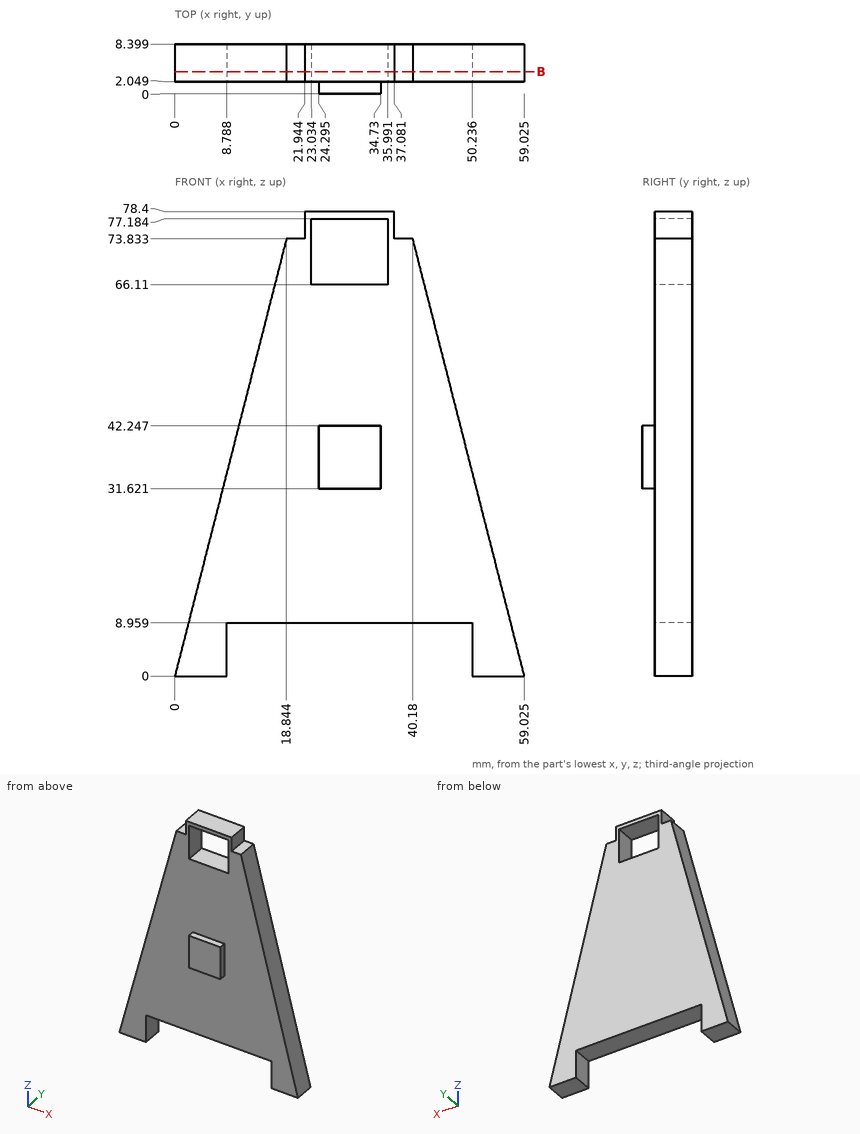
Check sheet for the drawn part. Datum: minimum x, y, z corner. Units: mm. Give positions to 0.01 mm unless a question says otherwise; leave off trailing zeros. Loops run counter-clockwise (first coordinate to the right, second up) from the corner with the lowest first, then second, coordinate; pieces in that order, holes last. Notation, with made-up numbers: (-15.5, 86.25) - (8.5, 86.25) arc R23 ccw to (8.5, 122.25) - close; hole circle Ø8 at (85.5, 31.25). An arc over 180 degrees is marked (long way). Write each question's results on one line, items separated by ' | '.
1) Depth check by flat-ended pin: P1, Ø2.5, axis at y = 3.5, z = 77, coming from the -X side; P2, Ø3.5, axis at y = 5.5, z = 76, coming from the +X side; P3, Ø1.6, axis at x = 29.5, y = 1.5, coming from the -Z side; P4, Ø17.5, axis at x = 26.5, z = 45, coming from the -Y side. Enter the tip coordinate at first touch or a pass-through.
Solution:
P1: x = 21.94 | P2: x = 37.08 | P3: z = 8.96 | P4: y = 0
2) Material ranges on L1, parallel to Z at x = 35, y = 5.75 (1 decimal); L2, parallel to Y at x = 4, z = 15; L3, parallel to Z at x = 40, y = 3.5, recorded low to high. Write a range as from..to.
Solution:
L1: 9..66.1, 77.2..78.4 | L2: 2.05..8.4 | L3: 8.96..73.83
3) Sectioned sample at B-B on y = 3.75. Record the boundary of the cut face in (x, z) (1 decimal).
Solution:
outline: (0, 0) - (8.8, 0) - (8.8, 9) - (50.2, 9) - (50.2, 0) - (59, 0) - (40.2, 73.8) - (37.1, 73.8) - (37.1, 78.4) - (21.9, 78.4) - (21.9, 73.8) - (18.8, 73.8) - close; hole (23, 66.1) - (36, 66.1) - (36, 77.2) - (23, 77.2) - close
